Read the model definition and answer for the solid it produces. Units are mm, in the model's axes. A direction names the side the tool comes from. Coordinates: 2 decimals unless noted, no trailing zeros. Write each loop counter-clockwise with the first axis right and the second up, starting at its lowest first coordinate (ties: lowest second). Pieces come first, ordered by that corner, then holes. Notation, with made-up numbers: (-27.75, -26) -> (25.25, -26) arc R25 ccw to (25.25, -10) -> close; hole circle Ø10 at (-29, 62). An arc over 180 degrees is marked (long way). Use CSV: the item, a comma, the result in double quotes. Start each with the question number.
from build123d import *

# Parameters (mm, degrees)
F0_W     = 609.6
F0_H     = 558.8
F0_W_2   = 571.5
F0_H_2   = 508
F1_DEPTH = 609.6
F2_W     = 571.5
F2_H     = 508
F3_DEPTH = 609.601
F4_W     = 596.9
F4_H     = 596.9
F5_DEPTH = 25.4
F6_W     = 546.1
F6_H     = 546.1
F7_DEPTH = 6.35
F8_W     = 571.5
F8_H     = 571.5
F9_DEPTH = 19.05


with BuildPart() as f1:
    # F0 (on Front) → F1 (new body)
    with BuildSketch(Plane.XZ):
        with Locations((304.8, 279.4)):
            Rectangle(F0_W, F0_H)
        with Locations((304.8, 273.05)):
            Rectangle(F0_W_2, F0_H_2, mode=Mode.SUBTRACT)
    extrude(amount=F1_DEPTH)

    # F2 (on face) → F3 (cut, through all)
    with BuildSketch(Plane.YZ.offset(609.6)):
        with Locations((-304.8, 273.05)):
            Rectangle(F2_W, F2_H)
    extrude(amount=-F3_DEPTH, mode=Mode.SUBTRACT)

    # F4 (on face) → F5 (cut)
    with BuildSketch(Plane.XY.offset(558.8)):
        with Locations((304.8, -304.8)):
            Rectangle(F4_W, F4_H)
    extrude(amount=-F5_DEPTH, mode=Mode.SUBTRACT)

    # F6 (on face) → F7 (cut, through all)
    with BuildSketch(Plane.XY.offset(533.4)):
        with Locations((304.8, -304.8)):
            Rectangle(F6_W, F6_H)
    extrude(amount=-F7_DEPTH, mode=Mode.SUBTRACT)

    # F8 (on face) → F9 (cut, through all)
    with BuildSketch(Plane.XY.offset(19.05)):
        with Locations((304.8, -304.8)):
            Rectangle(F8_W, F8_H)
    extrude(amount=-F9_DEPTH, mode=Mode.SUBTRACT)


solid = f1.part
1) Section C-C, the plane z = 258 is taken. Give the vertices of the cut face in (x, y).
2) This flat-tipped pin is pushed along its axis until it touches: pin 1 (9.5 mm diameter, centred on x = 229.5, y = -11.5, fed in from +Z). Where does it stop, or does it pass through?
3) Section B-B, the plane x = 517 is taken. Give the vertices of the cut face in (y, z).
4) Find the intervals of material crossed by line 1 along X through (y, z) = (-71.5, 533.5); line 2 along X through (y, z) = (-407.5, 531), in increasing order.
5) The mould has two halves that part along Y. Classify faces 1 (the face through (6.35, -309, 546)), 2 (the face through (303, 0, 529)), 3 (the face through (281, -597, 0)), 4 (the face through (281, -591, 533.4)): pulls with the +Y half, pulls with the -Y half, needs draft (parallel to the pull), parting line crosses it, or undercut.
6) Which of the six approach directions +Z, -Z, +X, -X, +Y, -Y give full straight-line access (tool end or side, diameter ignored) to faces 5 (the face through (301, -603.25, 546)), 6 (the face through (600, -590.55, 269)), 7 (the face through (301, -590.55, 10)), 8 (the face through (19.05, -600, 269))?
7) Section A-A, the plane y = -59 is taken. Give the vertices of the cut face in (x, z).
The answers:
1,outline,"(0, -609.6) -> (19.05, -609.6) -> (19.05, -590.55) -> (0, -590.55) -> close; (0, -19.05) -> (19.05, -19.05) -> (19.05, 0) -> (0, 0) -> close; (590.55, -609.6) -> (609.6, -609.6) -> (609.6, -590.55) -> (590.55, -590.55) -> close; (590.55, -19.05) -> (609.6, -19.05) -> (609.6, 0) -> (590.55, 0) -> close"
2,pin 1,"stops at z = 533.4"
3,outline,"(-609.6, 0) -> (-590.55, 0) -> (-590.55, 19.05) -> (-609.6, 19.05) -> close; (-609.6, 527.05) -> (-577.85, 527.05) -> (-577.85, 533.4) -> (-603.25, 533.4) -> (-603.25, 558.8) -> (-609.6, 558.8) -> close; (-31.75, 527.05) -> (0, 527.05) -> (0, 558.8) -> (-6.35, 558.8) -> (-6.35, 533.4) -> (-31.75, 533.4) -> close; (-19.05, 0) -> (0, 0) -> (0, 19.05) -> (-19.05, 19.05) -> close"
4,line 1,"x = 0 to 6.35, 603.25 to 609.6"
4,line 2,"x = 0 to 31.75, 577.85 to 609.6"
5,face 1,"undercut"
5,face 2,"pulls with the +Y half"
5,face 3,"needs draft"
5,face 4,"undercut"
6,face 5,"+Z"
6,face 6,"+X, -X"
6,face 7,"-Z"
6,face 8,"+Y, -Y"
7,outline,"(0, 0) -> (19.05, 0) -> (19.05, 19.05) -> (0, 19.05) -> close; (0, 527.05) -> (31.75, 527.05) -> (31.75, 533.4) -> (6.35, 533.4) -> (6.35, 558.8) -> (0, 558.8) -> close; (577.85, 527.05) -> (609.6, 527.05) -> (609.6, 558.8) -> (603.25, 558.8) -> (603.25, 533.4) -> (577.85, 533.4) -> close; (590.55, 0) -> (609.6, 0) -> (609.6, 19.05) -> (590.55, 19.05) -> close"
